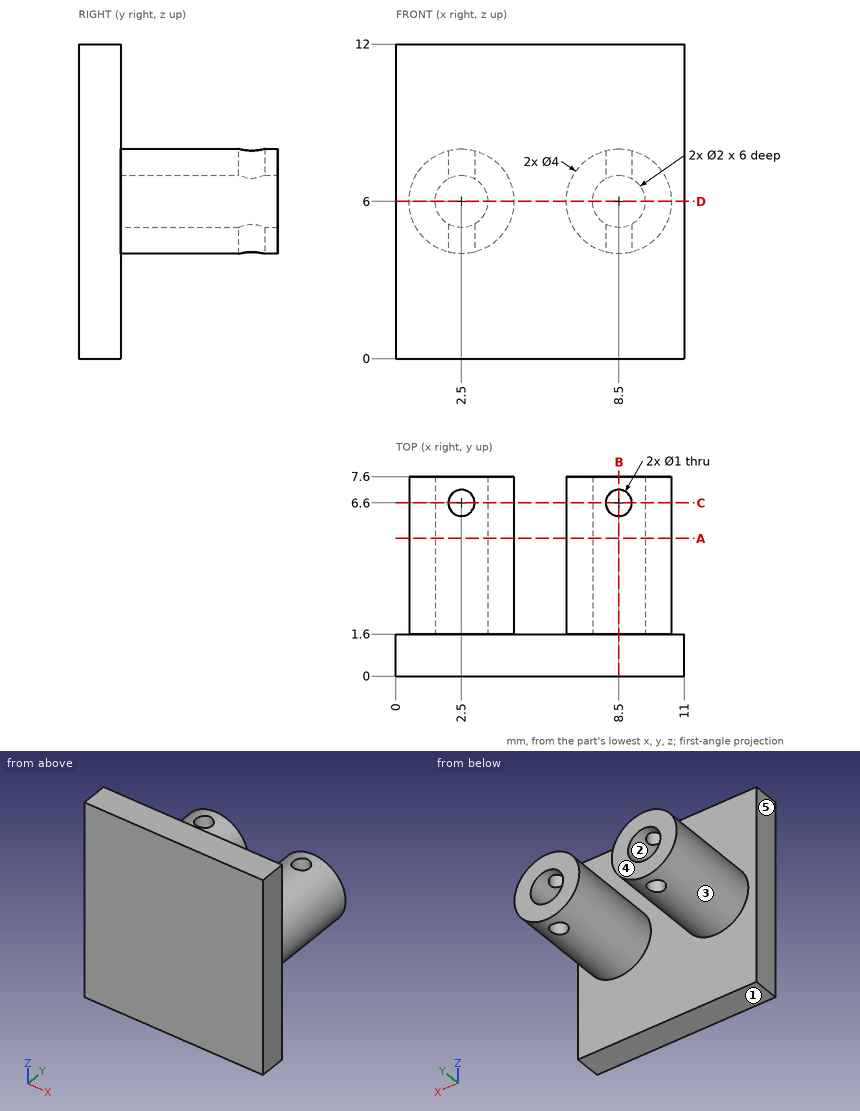
Study the drawing (mm; zero at the part's minimum x, y, z) and answer. A direction names the side the tool comes from. Give positions to 0.01 mm unless a question says otherwise; leave off trailing zeros. Loops run counter-clockwise (first coordinate to the right, second up) from the corner with the lowest first, then second, coordinate; pieces in that order, holes last. Notation, with made-up numbers: M 19.25,78.5 L 76.25,78.5 A28 ccw 76.25,99.5 Z; hole C 27,-30.5 d9. An arc over 180 degrees is marked long. Answer as CSV lines item,"result".
Item 1: Given pin 1 Ø4 at (x, z) = (5.5, 9) entering from +Y; pin 2 Ø3 at (x, y) = (2.5, 6.5) entering from +Z; pin 3 Ø2 at (y, z) = (1, 10) entering from -X, each flat-ended and moving along its own axis, determine where each tip first touches the part or whether it passes through.
Values follow:
pin 1,"stops at y = 1.6"
pin 2,"stops at z = 8"
pin 3,"stops at x = 0"
Item 2: Which of the six approach directions +Z, -Z, +X, -X, +Y, -Y give full straight-line access (tool end or side, diameter ignored) to the marked faces 1 and 2?
Values follow:
face 1,"-Z, +X, -X, +Y, -Y"
face 2,"+Y"
Item 3: The part is cut by section D-D (z = 6). Give the vertices of the cut face in (x, y).
Values follow:
outline,"M 0,0 L 11,0 L 11,1.6 L 10.5,1.6 L 10.5,7.6 L 9.5,7.6 L 9.5,1.6 L 7.5,1.6 L 7.5,7.6 L 6.5,7.6 L 6.5,1.6 L 4.5,1.6 L 4.5,7.6 L 3.5,7.6 L 3.5,1.6 L 1.5,1.6 L 1.5,7.6 L 0.5,7.6 L 0.5,1.6 L 0,1.6 Z"
Item 4: The part is cut by section A-A (y = 5.25). Give the vertices of the cut face in (x, z).
Values follow:
outline,"C 2.5,6 d4; C 8.5,6 d4; hole C 2.5,6 d2; hole C 8.5,6 d2"
Item 5: The part is cut by section B-B (x = 8.5). Give the vertices of the cut face in (y, z).
Values follow:
outline,"M 0,0 L 1.6,0 L 1.6,4 L 6.1,4 L 6.1,5 L 1.6,5 L 1.6,7 L 6.1,7 L 6.1,8 L 1.6,8 L 1.6,12 L 0,12 Z; M 7.1,4 L 7.6,4 L 7.6,5 L 7.1,5 Z; M 7.1,7 L 7.6,7 L 7.6,8 L 7.1,8 Z"
Item 6: Straight lines are drawn through the part: line 1 along X through (y, z) = (5.75, 6); line 2 along X through (y, z) = (6.6, 4.35); line 3 along Y through (x, z) = (6.75, 10.5). For each, find the intervals that lie inside material, in ascending order. Write a range as [from, to].
Values follow:
line 1,"x = [0.5, 1.5], [3.5, 4.5], [6.5, 7.5], [9.5, 10.5]"
line 2,"x = [1.37, 2], [3, 3.63], [7.37, 8], [9, 9.63]"
line 3,"y = [0, 1.6]"
Item 7: The mould has two halves that part along X. Classify the marked faces 3, 4 and 5: released by +X, released by -X, zero draft, split by the parting line, or undercut.
Values follow:
face 3,"undercut"
face 4,"zero draft"
face 5,"released by -X"
Item 8: The part is cut by section C-C (y = 6.6). Give the vertices of the cut face in (x, z).
Values follow:
outline,"M 2,4.06 L 2,5.13 A1 cw 2,6.87 L 2,7.94 A2 ccw Z; M 3,4.06 A2 ccw 3,7.94 L 3,6.87 A1 cw 3,5.13 Z; M 8,4.06 L 8,5.13 A1 cw 8,6.87 L 8,7.94 A2 ccw Z; M 9,4.06 A2 ccw 9,7.94 L 9,6.87 A1 cw 9,5.13 Z"
